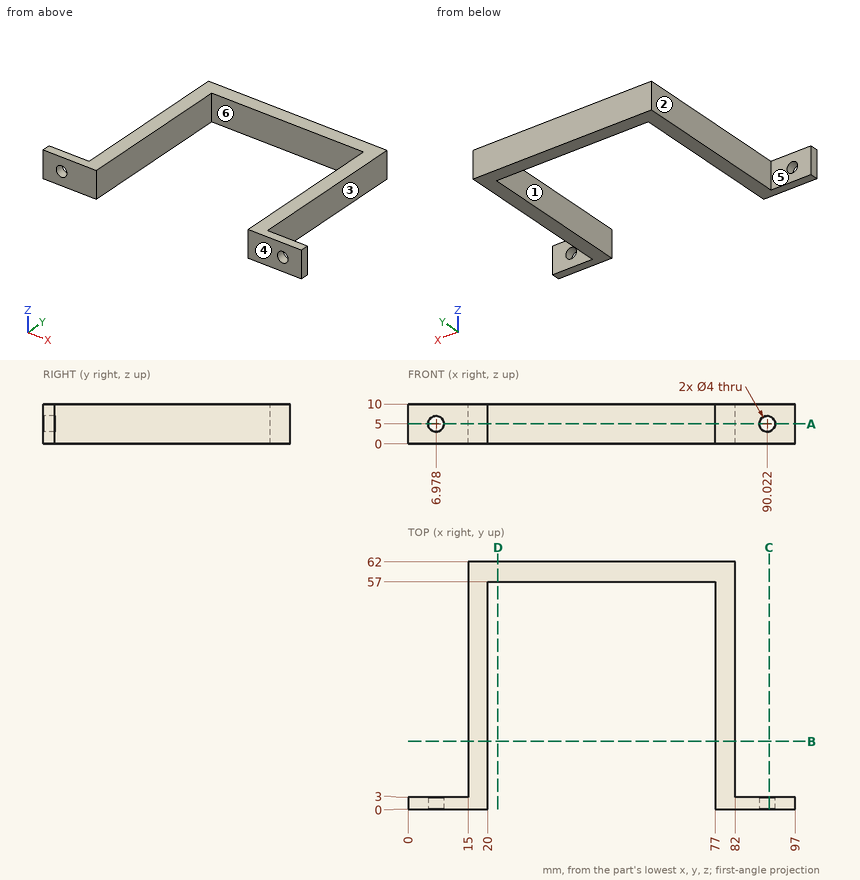
Design review of the part shown in the three views and the two pictorial views. Dimensions are in mm from the part's minimum x, y and z. A direction names the side the tool comes from. Give positions to 0.01 mm unless a question says otherwise; leave off trailing zeros. Loops run counter-clockwise (first coordinate to the right, second up) from the corner with the lowest first, then second, coordinate; pieces in that order, holes last. Notation, with made-up numbers: (22, -16.5) - (66, -16.5) arc R24 cw to (66, 5.5) - close; hole circle Ø1 at (5, -16.5). An arc over 180 degrees is marked (long way). Answer as a JSON object with one key per item and string values.
Q1. Insertion check: pin 1 (3 mm diameter, centred on y = 24.5, z = 6, fed in from +X); pin 2 (4 mm diameter, centred on y = 39.5, z = 7, fed in from -X); pin 3 (1 mm diameter, centred on x = 50.5, z = 9, fed in from -Y). Each pin has a flat end and moves straight along its axis. Give the tip position at first contact, or say it passes through.
Worked out:
{"pin 1": "stops at x = 82", "pin 2": "stops at x = 15", "pin 3": "stops at y = 57"}
Q2. Add section C-C on x = 90.5. State the section outline as (y, z) points.
Worked out:
{"outline": "(0, 0) - (3, 0) - (3, 3.06) - (0, 3.06) - close; (0, 6.94) - (3, 6.94) - (3, 10) - (0, 10) - close"}
Q3. Mouldability with a two-part tool opening along X and no side actions: class the marked faces 1, 2 and 3 as +X half, -X half, draft (parallel to the pull), parting line (faces both ways), or undercut.
Worked out:
{"face 1": "undercut", "face 2": "-X half", "face 3": "+X half"}
Q4. For the marked faces 4, 5 and 6, list the 3-axis set-ups (+Z, -Z, +X, -X, +Y, -Y) from which the entire face can be reached by the end or side of a thin tool; tool diameter is ignored.
Worked out:
{"face 4": "+Z, -Z, +X, -X, -Y", "face 5": "+Z, -Z, -X, +Y", "face 6": "+Z, -Z, -Y"}
Q5. To check wall thickness, follow line 1 along X through (y, z) = (2, 5); line 2 along X through (y, z) = (25, 3); line 3 along Y through (x, z) = (58, 6.5). State the ranges of each line that lie inside material, in increasing order.
Worked out:
{"line 1": "x = 0 to 4.98, 8.98 to 20, 77 to 88.02, 92.02 to 97", "line 2": "x = 15 to 20, 77 to 82", "line 3": "y = 57 to 62"}
Q6. Add section A-A on z = 5. State the section outline as (x, y) points.
Worked out:
{"outline": "(0, 0) - (4.98, 0) - (4.98, 3) - (0, 3) - close; (8.98, 0) - (20, 0) - (20, 57) - (77, 57) - (77, 0) - (88.02, 0) - (88.02, 3) - (82, 3) - (82, 62) - (15, 62) - (15, 3) - (8.98, 3) - close; (92.02, 0) - (97, 0) - (97, 3) - (92.02, 3) - close"}
Q7. Add section D-D on x = 22.5. State the section outline as (y, z) points.
Worked out:
{"outline": "(57, 0) - (62, 0) - (62, 10) - (57, 10) - close"}
Q8. Add section B-B on y = 17. State the section outline as (x, z) points.
Worked out:
{"outline": "(15, 0) - (20, 0) - (20, 10) - (15, 10) - close; (77, 0) - (82, 0) - (82, 10) - (77, 10) - close"}
